from build123d import *

# Parameters (mm, degrees)
SKETCH2_R            = 1.1
SKETCH2_R_2          = 1.2
BOSS_EXTRUDE4_DEPTH  = 3
FILLET2_R            = 9
FILLET3_R            = 4.2
CUT_EXTRUDE1_DEPTH   = 17
FILLET4_R            = 3
FILLET5_R            = 2
SKETCH6_R            = 1.2
BOSS_EXTRUDE6_DEPTH  = 3
FILLET6_R            = 1
FILLET4_OF_MIRROR1_R = 3
FILLET5_OF_MIRROR1_R = 2


with BuildPart() as part:
    # Sketch2 → Boss-Extrude4 (new body)
    # profile 1 of 7: a face of its own
    with BuildSketch(Plane.XY):
        with BuildLine():
            ThreePointArc((27, 110), (20.291796068, 111.583592135), (15, 116))
            Line((15, 116), (15, 110))
            Line((15, 110), (27, 110))
        make_face()
    # profile 2 of 7: a face of its own
    with BuildSketch(Plane.XY):
        with BuildLine():
            ThreePointArc((76, 116), (70.708203932, 111.583592135), (64, 110))
            Line((64, 110), (76, 110))
            Line((76, 110), (76, 116))
        make_face()
    # profile 3 of 7: a face of its own
    with BuildSketch(Plane.XY):
        Polygon((20, 0), (0, 0), (0, 25), (7, 25), (7, 116), (15, 116), (15, 110), (76, 110), (76, 116), (84, 116), (84, 25), (91, 25), (91, 0), (71, 0), (71, 6), (20, 6), align=None)
        with Locations((86.75, 22.3)):
            Circle(SKETCH2_R, mode=Mode.SUBTRACT)
        with Locations((21.4, 84)):
            Circle(SKETCH2_R_2, mode=Mode.SUBTRACT)
        with Locations((69.6, 82.7)):
            Circle(SKETCH2_R_2, mode=Mode.SUBTRACT)
        with Locations((54.4, 31.9)):
            Circle(SKETCH2_R_2, mode=Mode.SUBTRACT)
        with Locations((26.5, 31.9)):
            Circle(SKETCH2_R_2, mode=Mode.SUBTRACT)
        with Locations((4.25, 22.3)):
            Circle(SKETCH2_R, mode=Mode.SUBTRACT)
        with Locations((4.25, 4.3)):
            Circle(SKETCH2_R, mode=Mode.SUBTRACT)
        with Locations((86.75, 4.3)):
            Circle(SKETCH2_R, mode=Mode.SUBTRACT)
        with BuildLine():
            ThreePointArc((30, 74), (28.5, 75.5), (27, 74))
            Line((27, 74), (27, 56))
            ThreePointArc((27, 56), (28.5, 54.5), (30, 56))
            Line((30, 56), (30, 74))
        make_face(mode=Mode.SUBTRACT)
        with BuildLine():
            Line((61, 56), (61, 74))
            ThreePointArc((61, 74), (62.5, 75.5), (64, 74))
            Line((64, 74), (64, 56))
            ThreePointArc((64, 56), (62.5, 54.5), (61, 56))
        make_face(mode=Mode.SUBTRACT)
    # profile 4 of 7: a face of its own
    with BuildSketch(Plane.XY):
        with BuildLine():
            ThreePointArc((7, 37.124355653), (5.124355653, 30.124355653), (0, 25))
            Line((0, 25), (7, 25))
            Line((7, 25), (7, 37.124355653))
        make_face()
    # profile 5 of 7: a face of its own
    with BuildSketch(Plane.XY):
        with BuildLine():
            Line((84, 25), (91, 25))
            ThreePointArc((91, 25), (85.875644326, 30.124355689), (84, 37.124355736))
            Line((84, 37.124355736), (84, 25))
        make_face()
    # profile 6 of 7: a face of its own
    with BuildSketch(Plane.XY):
        with BuildLine():
            Line((71, 6), (63.254033308, 6))
            ThreePointArc((63.254033308, 6), (68.153012793, 4.32455532), (71, 0))
            Line((71, 0), (71, 6))
        make_face()
    # profile 7 of 7: a face of its own
    with BuildSketch(Plane.XY):
        with BuildLine():
            Line((20, 6), (20, 0))
            ThreePointArc((20, 0), (22.846987207, 4.32455532), (27.745966692, 6))
            Line((27.745966692, 6), (20, 6))
        make_face()
    extrude(amount=BOSS_EXTRUDE4_DEPTH)

    # Fillet2
    fillet2_edges = [part.edges().sort_by_distance(p)[0] for p in [
        (15, 116, 1.5),
        (76, 116, 1.5),
        (71, 0, 1.5),
        (20, 0, 1.5),
    ]]
    fillet(fillet2_edges, radius=FILLET2_R)

    # Fillet3
    fillet3_edges = [part.edges().sort_by_distance(p)[0] for p in [
        (0, 0, 1.5),
        (0, 25, 1.5),
        (91, 25, 1.5),
        (91, 0, 1.5),
    ]]
    fillet(fillet3_edges, radius=FILLET3_R)

    # Sketch3 → Cut-Extrude1 (cut)
    with BuildSketch(Plane.XY.offset(3)):
        with BuildLine():
            ThreePointArc((21, 64), (18.954521952, 77.564659966), (13, 89.922962794))
            Line((13, 89.922962794), (13, 38.077037206))
            ThreePointArc((13, 38.077037206), (18.954521952, 50.435340034), (21, 64))
        make_face()
        with BuildLine():
            Line((28.5, 103), (45.5, 103))
            Line((45.5, 103), (45.5, 86))
            ThreePointArc((45.5, 86), (33.47918472, 90.97918472), (28.5, 103))
        make_face()
        with BuildLine():
            Line((45.5, 12), (45.5, 29))
            ThreePointArc((45.5, 29), (33.47918472, 24.02081528), (28.5, 12))
            Line((28.5, 12), (45.5, 12))
        make_face()
    cut_extrude1 = extrude(amount=-CUT_EXTRUDE1_DEPTH, mode=Mode.SUBTRACT)

    # Fillet4
    fillet4_edges = [part.edges().sort_by_distance(p)[0] for p in [
        (28.5, 103, 1.5),
        (28.5, 12, 1.5),
    ]]
    fillet(fillet4_edges, radius=FILLET4_R)

    # Fillet5
    fillet5_edges = [part.edges().sort_by_distance(p)[0] for p in [
        (13, 38.077037206, 1.5),
        (13, 89.922962794, 1.5),
    ]]
    fillet(fillet5_edges, radius=FILLET5_R)

    # Sketch6 → Boss-Extrude6 (add)
    with BuildSketch(Plane.XY.offset(3)):
        with BuildLine():
            ThreePointArc((4.386675042, 113.273568309), (4.244027857, 112.706113443), (3.85, 112.273568309))
            Line((3.85, 112.273568309), (7, 112.273568309))
            Line((7, 112.273568309), (7, 116))
            ThreePointArc((7, 116), (4.500310829, 115.51828106), (2.358656251, 114.142121636))
            ThreePointArc((2.358656251, 114.142121636), (3.659103582, 114.376659998), (4.386675042, 113.273568309))
        make_face()
        with Locations((3.186675042, 113.273568309)):
            Circle(SKETCH6_R)
        with Locations((3.186675042, 106.273568309)):
            Circle(SKETCH6_R)
        with BuildLine():
            ThreePointArc((4.386675042, 106.273568309), (3.659103582, 105.17047662), (2.358656251, 105.405014982))
            ThreePointArc((2.358656251, 105.405014982), (4.500310829, 104.028855558), (7, 103.547136618))
            Line((7, 103.547136618), (7, 107.273568309))
            Line((7, 107.273568309), (3.85, 107.273568309))
            ThreePointArc((3.85, 107.273568309), (4.244027857, 106.841023175), (4.386675042, 106.273568309))
        make_face()
        with Locations((3.186675042, 73.273568309)):
            Circle(SKETCH6_R)
        with BuildLine():
            ThreePointArc((4.386675042, 73.273568309), (4.244027857, 72.706113443), (3.85, 72.273568309))
            Line((3.85, 72.273568309), (7, 72.273568309))
            Line((7, 72.273568309), (7, 76))
            ThreePointArc((7, 76), (4.500310865, 75.518281074), (2.358656308, 74.14212169))
            ThreePointArc((2.358656308, 74.14212169), (3.659103618, 74.376659983), (4.386675042, 73.273568309))
        make_face()
        with Locations((3.186675042, 66.273568309)):
            Circle(SKETCH6_R)
        with BuildLine():
            ThreePointArc((4.386675042, 66.273568309), (3.659103622, 65.170476637), (2.358656313, 65.405014923))
            ThreePointArc((2.358656313, 65.405014923), (4.500310869, 64.028855542), (7, 63.547136618))
            Line((7, 63.547136618), (7, 67.273568309))
            Line((7, 67.273568309), (3.85, 67.273568309))
            ThreePointArc((3.85, 67.273568309), (4.244027857, 66.841023175), (4.386675042, 66.273568309))
        make_face()
    boss_extrude6 = extrude(amount=-BOSS_EXTRUDE6_DEPTH)

    # Fillet6
    fillet6_edges = [part.edges().sort_by_distance(p)[0] for p in [
        (3.85, 112.273568309, 1.5),
        (3.85, 107.273568309, 1.5),
        (3.85, 72.273568309, 1.5),
        (3.85, 67.273568309, 1.5),
    ]]
    fillet(fillet6_edges, radius=FILLET6_R)

    # Mirror1: Cut-Extrude1, Boss-Extrude6 across plane
    add(cut_extrude1.mirror(Plane(origin=(45.5, 0, -14), x_dir=(0, 0, 1), z_dir=(-1, 0, 0))), mode=Mode.SUBTRACT)
    add(boss_extrude6.mirror(Plane(origin=(45.5, 0, -14), x_dir=(0, 0, 1), z_dir=(-1, 0, 0))))

    # Fillet4 of Mirror1
    fillet4_of_mirror1_edges = [part.edges().sort_by_distance(p)[0] for p in [
        (62.5, 103, 1.5),
        (62.5, 12, 1.5),
    ]]
    fillet(fillet4_of_mirror1_edges, radius=FILLET4_OF_MIRROR1_R)

    # Fillet5 of Mirror1
    fillet5_of_mirror1_edges = [part.edges().sort_by_distance(p)[0] for p in [
        (78, 38.077037206, 1.5),
        (78, 89.922962794, 1.5),
    ]]
    fillet(fillet5_of_mirror1_edges, radius=FILLET5_OF_MIRROR1_R)


solid = part.part
Design review of the part built by this model. Coordinates are the model's own, in mm. A direction names the side the tool comes from. Round coordinates to 2 decimals unless told otherwise and drop trailing zeros. Loops run counter-clockwise (first coordinate to the right, second up) from the corner with the lowest first, then second, coordinate; pieces in that order, holes last. Notation, with made-up numbers: (19, -19) - (51, -19) arc R16 ccw to (51, -8) - close; hole circle Ø2 at (22.25, -11.75). An arc over 180 degrees is marked (long way). One line per item, written item: value. Start each with the question number.
1) Consider section A-A on x = 38.5. Give the boundary of the cut face in (y, z), then the cut area to 3 significant figures.
2) Insertion check: pin 1 Ø1.5 at (x, z) = (85.5, 1) entering from +Y; pin 2 Ø1.5 at (y, z) = (38, 1) entering from -X; pin 3 Ø0.9 at (y, z) = (92.5, 2) entering from +X. Each pin has a flat end and moves straight along its axis. Give the tip position at first contact, or say it passes through.
3) Consider section C-C on z = 1.85. Give the number of separate pieces and of enclosed holes in the cut face, then the cut area to 3 significant figures.
4) Draft analysis for pull direction Y (two halves, no side actions). For faces 1 (the cylindrical face through (0.414, 24.596, 1.521)), 2 (the flat face through (82, 0, 1)), 3 (the cylindrical face through (4.47, 104.04, 1.52)), state which applies: +Y half, -Y half, draft (parallel to the pull), parting line (faces both ways), or undercut.
5) For faces 4 (the flat face through (46, 6, 1)), 5 (the cylindrical face through (1.26, 1.2, 1.52)), 6 (the cylindrical face through (69.374, 110.996, 1.479)), 7 (the cylindrical face through (5.621, 31.065, 1.479)), 8 (the cylindrical face through (62.5, 75.5, 1.5)), list the 3-axis set-ups (+Z, -Z, +X, -X, +Y, -Y) from which the entire face can be reached by the end or side of a thin tool; tool diameter is ignored.
6) Consider section B-B on y = 59.5. Give the boundary of the cut face in (x, z), then the cut area to 3 significant figures.
7) Consider section D-D on y = 31.9. Give the boundary of the cut face in (x, z), then the cut area to 3 significant figures.
8) To check wall thickness, follow L1, parallel to X at y = 66, z = 1.95; L2, parallel to X at y = 81, z = 2.6; L3, parallel to Y at x = 37, z = 0.8. State the ranges of each line that lie inside material, in increasing order. Write a range as from..to.
Reported:
1. outline: (6, 0) - (12, 0) - (12, 3) - (6, 3) - close; (27.49, 0) - (87.51, 0) - (87.51, 3) - (27.49, 3) - close; (103, 0) - (110, 0) - (110, 3) - (103, 3) - close
1. area: 219 mm^2
2. pin 1: stops at y = 115.96
2. pin 2: stops at x = 7
2. pin 3: stops at x = 84
3. separate pieces: 1
3. enclosed holes: 14
3. area: 7,260 mm^2
4. face 1: +Y half
4. face 2: -Y half
4. face 3: undercut
5. face 4: +Z, -Z, -Y
5. face 5: +Z, -Z, -X, -Y
5. face 6: +Z, -Z, +Y
5. face 7: +Z, -Z, -X
5. face 8: +Z, -Z
6. outline: (7, 0) - (13, 0) - (13, 3) - (7, 3) - close; (20.78, 0) - (27, 0) - (27, 3) - (20.78, 3) - close; (30, 0) - (61, 0) - (61, 3) - (30, 3) - close; (64, 0) - (70.22, 0) - (70.22, 3) - (64, 3) - close; (78, 0) - (84, 0) - (84, 3) - (78, 3) - close
6. area: 166 mm^2
7. outline: (5.99, 0) - (25.3, 0) - (25.3, 3) - (5.99, 3) - close; (27.7, 0) - (53.2, 0) - (53.2, 3) - (27.7, 3) - close; (55.6, 0) - (85.01, 0) - (85.01, 3) - (55.6, 3) - close
7. area: 223 mm^2
8. L1: x = 2.02..13, 20.96..27, 30..61, 64..70.04, 78..88.98
8. L2: x = 7..13, 17.74..73.26, 78..84
8. L3: y = 6..12, 26.72..88.28, 103..110
